```python
from build123d import *

# Parameters (mm, degrees)
F0_W      = 2000
F0_H      = 200
F1_DEPTH  = 30
F2_W      = 10
F2_H      = 10
F3_DEPTH  = 2000
F5_R      = 3
F6_DEPTH  = 30
F7_R      = 3
F8_DEPTH  = 30
F4_W      = 10
F4_H      = 10
F9_DEPTH  = 2000
F11_D     = 5.1054
F11_DEPTH = 30
F11_TIP   = 1.5338169022
F13_D     = 5.1054
F13_DEPTH = 30
F13_TIP   = 1.5338169022


with BuildPart() as f1:
    # F0 (on Right) → F1 (new body)
    with BuildSketch(Plane.YZ):
        Rectangle(F0_W, F0_H)
    extrude(amount=F1_DEPTH)

    # F2 (on face) → F3 (join)
    with BuildSketch(Plane.XZ.offset(1000)):
        with Locations((5, 105)):
            Rectangle(F2_W, F2_H)
    extrude(amount=-F3_DEPTH)

    # F5 (on face) → F6 (join)
    with BuildSketch(Plane(origin=(0, 1000, 0), x_dir=(-1, 0, 0), z_dir=(0, 1, 0))):
        with Locations((-15, -50)):
            Circle(F5_R)
        with Locations((-15, 50.2506281447)):
            Circle(F5_R)
    extrude(amount=F6_DEPTH)

    # F7 (on face) → F8 (join)
    with BuildSketch(Plane.XZ.offset(1000)):
        with Locations((15, 50)):
            Circle(F7_R)
        with Locations((15, -50)):
            Circle(F7_R)
    extrude(amount=F8_DEPTH)

    # F4 (on face) → F9 (join)
    with BuildSketch(Plane.XZ.offset(1000)):
        with Locations((25, 105)):
            Rectangle(F4_W, F4_H)
    extrude(amount=-F9_DEPTH)

    # F11
    with Locations(Plane.XZ.offset(1000)):
        with Locations((15, 0)):
            Hole(F11_D / 2, depth=F11_DEPTH)
            with Locations((0, 0, -(F11_DEPTH + F11_TIP / 2))):  # 118° drill point
                Cone(0, F11_D / 2, F11_TIP, mode=Mode.SUBTRACT)

    # F13
    with Locations(Plane(origin=(0, 1000, 0), x_dir=(-1, 0, 0), z_dir=(0, 1, 0))):
        with Locations((-15, 0)):
            Hole(F13_D / 2, depth=F13_DEPTH)
            with Locations((0, 0, -(F13_DEPTH + F13_TIP / 2))):  # 118° drill point
                Cone(0, F13_D / 2, F13_TIP, mode=Mode.SUBTRACT)


solid = f1.part
```
The listing builds one solid part. Answer for the finished solid, in the listing's coordinates (mm). Coordinates: 2 decimals unless noted, no trailing zeros. Write each loop counter-clockwise with the first axis right and the second up, starting at its lowest first coordinate (ties: lowest second). Pieces come first, ordered by that corner, then holes.
Q1. Section B-B, the plane x = 5.5 is taken. Write down the section's boundary in (y, z), then the cut area to 3 significant figures.
Returned:
outline: (-1000, -100) - (1000, -100) - (1000, 110) - (-1000, 110) - close
area: 420,000 mm2
Q2. Given P1, Ø4.5, axis at x = 15, z = 0, coming from the +Y side; P2, Ø2, axis at x = 20.5, z = -4.5, coming from the -Y side; P3, Ø4.5, axis at x = 15, z = 0, coming from the -Y side, each flat-ended and moving along its own axis, determine where each tip first touches the part or whether it passes through.
Returned:
P1: stops at y = 969.82
P2: stops at y = -1000
P3: stops at y = -969.82
Q3. Find the intervals of material crossed by line 1 along X through (y, z) = (-976.5, 0); line 2 along Z through (x, y) = (15, -991.5); line 3 along Z through (x, y) = (14.25, 294), in increasing order.
Returned:
line 1: x = 0 to 12.45, 17.55 to 30
line 2: z = -100 to -2.55, 2.55 to 100
line 3: z = -100 to 100
Q4. Section A-A, the plane y = 472 is taken. Write down the section's boundary in (x, z).
Returned:
outline: (0, -100) - (30, -100) - (30, 110) - (20, 110) - (20, 100) - (10, 100) - (10, 110) - (0, 110) - close
